```python
from build123d import *

# Parameters (mm, degrees)
SALIENTE_EXTRUIR1_DEPTH = 0.1


with BuildPart() as part:
    # Model → Saliente-Extruir1 (new body)
    with BuildSketch(Plane.XY):
        with BuildLine():
            Line((59.821558845, 14.577954318), (60.272695606, 14.399362661))
            ThreePointArc((60.272695606, 14.399362661), (60.398521137, 15.595766769), (60.551460532, 16.789007899))
            Line((60.551460532, 16.789007899), (51.49198027, 20.375387298))
            Line((51.49198027, 20.375387298), (38.316142065, 16.736158757))
            Line((38.316142065, 16.736158757), (25.140426213, 20.375830252))
            Line((25.140426213, 20.375830252), (16.080825387, 16.789755425))
            ThreePointArc((16.080825387, 16.789755425), (16.233724667, 15.596509154), (16.359509975, 14.400100817))
            Line((16.359509975, 14.400100817), (16.807003209, 14.577232707))
            Line((16.807003209, 14.577232707), (25.140342166, 17.875830254))
            Line((25.140342166, 17.875830254), (38.316058018, 14.236158759))
            Line((38.316058018, 14.236158759), (51.49198027, 17.875387298))
            Line((51.49198027, 17.875387298), (59.821558845, 14.577954318))
        make_face()
    extrude(amount=SALIENTE_EXTRUIR1_DEPTH)


solid = part.part
```
Build history of the part. All positions in model axes, mm. Round coordinates to 2 decimals unless told otherwise and drop trailing zeros. Loops run counter-clockwise (first coordinate to the right, second up) from the corner with the lowest first, then second, coordinate; pieces in that order, holes last.
Item 1: Drill centre lines: line 1 along Y through (x, z) = (25.5, 0.05); line 2 along Y through (x, z) = (45, 0.05). Where is each one in solid material? Low to high.
Item 2: Saw through at A-A (y = 16). List the corners of the cut face in (x, z), then the cut area to 3 significant figures.
Item 3: Saw through at C-C (y = 18.25). List the corners of the cut face in (x, z), then the cut area to 3 significant figures.
Item 4: Saw through at B-B (z = 0.05). List the corners of the cut face in (x, y), then the cut area to 3 significant figures.
Item 5: Saw through at D-D (x = 49). List the corners of the cut face in (y, z).
Worked answers:
1. line 1: y = 17.78 to 20.28
1. line 2: y = 16.08 to 18.58
2. outline: (16.19, 0) - (20.4, 0) - (20.4, 0.1) - (16.19, 0.1) - close; (31.93, 0) - (44.7, 0) - (44.7, 0.1) - (31.93, 0.1) - close; (56.23, 0) - (60.45, 0) - (60.45, 0.1) - (56.23, 0.1) - close
2. area: 2.12 mm2
3. outline: (19.77, 0) - (32.84, 0) - (32.84, 0.1) - (19.77, 0.1) - close; (43.8, 0) - (56.86, 0) - (56.86, 0.1) - (43.8, 0.1) - close
3. area: 2.61 mm2
4. outline: (16.08, 16.79) arc R53.02 cw to (16.36, 14.4) - (25.14, 17.88) - (38.32, 14.24) - (51.49, 17.88) - (60.27, 14.4) arc R53.02 cw to (60.55, 16.79) - (51.49, 20.38) - (38.32, 16.74) - (25.14, 20.38) - close
4. area: 110 mm2
5. outline: (17.19, 0) - (19.69, 0) - (19.69, 0.1) - (17.19, 0.1) - close
